Verification items for the finished model (mm, model axes). A direction names the side the tool comes from. Give positions to 0.01 mm unless a question says otherwise; leave off trailing zeros. Write each loop counter-clockwise with the first axis right and the second up, starting at its lowest first coordinate (ties: lowest second). Pieces come first, ordered by that corner, then holes. Notation, with made-up numbers: (13, 52.5) - (29, 52.5) arc R27 cw to (29, 75.5) - close; hole circle Ø2 at (-24.5, -14.5). An arc over 180 degrees is marked (long way). Answer as a JSON object with one key per item and string values. Group by question number.
Item 1: Scan lines: line 1 along Y through (x, z) = (0, -4.25); line 2 along Z through (x, y) = (0, -0.8); line 3 along Y through (x, z) = (-3.5, -6.5). Record each from-to range of solid material in increasing order. Write a range as [from, to].
Item 2: Sectioned sample at D-D, the plane x = -3.25. Record the boundary of the cut face in (y, z), and give its area (3 significant figures).
Item 3: Tool access check on faces 1 (the face through (5.7, -12, 0.5)), 2 (the face through (5.202, -12.507, 0.917)), 3 (the face through (2.6, -8.5, -4.5)). Record the directions out of +Z, -Z, +X, -X, +Y, -Y that give a thin tool (end or side, any length) a straight path to the whole face; none if there is none.
Item 4: Go/stop test with flat-tipped pins: pin 1 (2 mm diameter, centred on y = -8.5, z = 2, fed in from -X); pin 2 (1 mm diameter, centred on x = 0, y = -2.5, fed in from -Z); pin 3 (4 mm diameter, centred on y = -1.5, z = 5.5, fed in from +X); pin 4 (1.3 mm diameter, centred on x = 5, y = -10, fed in from +Z). Record where each tip stops, or that it passes through.
Item 5: Sectioned sample at B-B, the plane y = -5.75. Record the boundary of the cut face in (x, z), and give its area (3 significant figures).
Item 6: Sectioned sample at A-A, the plane x = 0. Record the boundary of the cut face in (y, z), and give its area (3 significant figures).
Item 7: Sectioned sample at C-C, the plane z = 4.25. Record the boundary of the cut face in (x, y).
Item 8: Draft check along Y on faces 4 (the face through (0.104, -4.01, 0.793)), 5 (the face through (4, -13, -3)), 6 (the face through (2, -12, -5)). Enter one of: +Y half, -Y half, draft (parallel to the pull), parting line (faces both ways), or undercut.
```python
from build123d import *

# Parameters (mm, degrees)
F0_R     = 7.5
F1_DEPTH = 5
F3_DEPTH = 8
F4_R     = 0.8
F5_DEPTH = 13.001
F6_R     = 0.8
F7_DEPTH = 12.5
F9_DEPTH = 1


with BuildPart() as f1:
    # F0 (on Front) → F1 (new body)
    with BuildSketch(Plane.XZ):
        Circle(F0_R)
    extrude(amount=F1_DEPTH)

    # F2 (on face) → F3 (join)
    with BuildSketch(Plane.XZ.offset(5)):
        with BuildLine():
            ThreePointArc((-2.9991336175, 0.0047529666), (-2.5960245368, 1.5020576249), (-1.4991373826, 2.5980762114))
            Line((-1.4991373826, 2.5980762114), (-3.7493530184, 6.4955640204))
            ThreePointArc((-3.7493530184, 6.4955640204), (-6.4938150879, 3.7523813244), (-7.499998494, 0.0047529666))
            Line((-7.499998494, 0.0047529666), (-2.9991336175, 0.0047529666))
        make_face()
        with BuildLine():
            ThreePointArc((3.0008588523, 0.0047529666), (2.6001262556, -1.4979414338), (1.5008626174, -2.5980762114))
            Line((1.5008626174, -2.5980762114), (3.7506469444, -6.4948169719))
            ThreePointArc((3.7506469444, -6.4948169719), (6.4965650956, -3.7476181714), (7.499998494, 0.0047529666))
            Line((7.499998494, 0.0047529666), (3.0008588523, 0.0047529666))
        make_face()
    extrude(amount=F3_DEPTH)

    # F4 (on face) → F5 (cut, through all)
    with BuildSketch(Plane(origin=(0, 0, 0), x_dir=(-1, 0, 0), z_dir=(0, 1, 0))):
        Circle(F4_R)
    extrude(amount=-F5_DEPTH, mode=Mode.SUBTRACT)

    # F6 (on Top) → F7 (cut, symmetric)
    with BuildSketch(Plane.XY):
        with Locations((0, -2.5)):
            Circle(F6_R)
    extrude(amount=F7_DEPTH, both=True, mode=Mode.SUBTRACT)

    # F8 (on face) → F9 (join)
    with BuildSketch(Plane.XZ.offset(13)):
        with BuildLine():
            ThreePointArc((2.9552858764, 0.520944533), (2.5989388287, -1.5), (1.0269230474, -2.8190778624))
            Line((1.0269230474, -2.8190778624), (2.5659127703, -7.0474173748))
            ThreePointArc((2.5659127703, -7.0474173748), (6.4953557229, -3.7497138602), (7.3860841572, 1.302213816))
            Line((7.3860841572, 1.302213816), (2.9552858764, 0.520944533))
        make_face()
        with BuildLine():
            Line((-7.386032135, -1.3025088485), (-2.9535606416, -0.520944533))
            ThreePointArc((-2.9535606416, -0.520944533), (-2.597213594, 1.5), (-1.0251978126, 2.8190778624))
            Line((-1.0251978126, 2.8190778624), (-2.5643893496, 7.0479718546))
            ThreePointArc((-2.5643893496, 7.0479718546), (-6.4950253213, 3.7502861326), (-7.386032135, -1.3025088485))
        make_face()
    extrude(amount=-F9_DEPTH)


solid = f1.part
```
Geometry check:
{
 "1": {"line 1": "[-5, -3.3], [-1.7, 0]", "line 2": "[-7.5, -0.8], [0.8, 7.5]", "line 3": "[-5, 0]"},
 "2": {"outline": "(-13, -0.57) - (-12, -0.57) - (-12, 0) - (-5, 0) - (-5, -6.76) - (0, -6.76) - (0, 6.76) - (-5, 6.76) - (-5, 5.63) - (-12, 5.63) - (-12, 6.76) - (-13, 6.76) - close", "area": "114 mm^2"},
 "3": {"face 1": "+Z, +X", "face 2": "+Z, -Y", "face 3": "-Z, -X"},
 "4": {"pin 1": "x = -7.43", "pin 2": "through", "pin 3": "x = 6.63", "pin 4": "z = 0"},
 "5": {"outline": "(-7.5, 0) - (-3, 0) arc R3 cw to (-1.5, 2.6) - (-3.75, 6.5) arc R7.5 ccw to start; (1.5, -2.6) - (3.75, -6.49) arc R7.5 ccw to (7.5, 0) - (3, 0) arc R3 cw to start", "area": "49.5 mm^2"},
 "6": {"outline": "(-5, -7.5) - (-3.3, -7.5) - (-3.3, -0.8) - (-5, -0.8) - close; (-5, 0.8) - (-3.3, 0.8) - (-3.3, 7.5) - (-5, 7.5) - close; (-1.7, -7.5) - (0, -7.5) - (0, -0.8) - (-1.7, -0.8) - close; (-1.7, 0.8) - (0, 0.8) - (0, 7.5) - (-1.7, 7.5) - close", "area": "45.6 mm^2"},
 "7": {"outline": "(-6.18, -13) - (-1.55, -13) - (-1.55, -12) - (-2.45, -12) - (-2.45, -5) - (6.18, -5) - (6.18, 0) - (-6.18, 0) - close; hole circle Ø1.6 at (0, -2.5)"},
 "8": {"face 4": "draft", "face 5": "-Y half", "face 6": "undercut"}
}
